```python
from build123d import *

# Parameters (mm, degrees)
F0_R     = 4
F0_W     = 8
F0_H     = 19
F1_DEPTH = 5
F0_H_2   = 1
F2_DEPTH = 8
F3_DEPTH = 5
F4_R     = 3
F5_SIZE2 = 2.99999
F5_SIZE  = 8.242422


# Not quite as in the source:
# - a fillet or chamfer is up to 0.001 mm smaller than in the source, because OpenCascade refuses the exact size


with BuildPart() as f1:
    # F0 (on Top) → F1 (new body)
    with BuildSketch(Plane.XY):
        Polygon((-15, 20), (-15, -25), (15, -25), (15, 20), (4, 20), (4, 1), (-4, 1), (-4, 20), align=None)
        with Locations((0, -15)):
            Circle(F0_R, mode=Mode.SUBTRACT)
        with Locations((0, 10.5)):
            Rectangle(F0_W, F0_H)
        with BuildLine():
            Line((-15, 25), (-15, 20))
            Line((-15, 20), (-4, 20))
            Line((-4, 20), (-4, 21))
            Line((-4, 21), (4, 21))
            Line((4, 21), (4, 20))
            Line((4, 20), (15, 20))
            Line((15, 20), (15, 25))
            Line((15, 25), (15, 31.3397459622))
            Line((15, 31.3397459622), (7.5, 27.0096189432))
            ThreePointArc((7.5, 27.0096189432), (0, 25), (-7.5, 27.0096189432))
            Line((-7.5, 27.0096189432), (-15, 31.3397459622))
            Line((-15, 31.3397459622), (-15, 25))
        make_face()
    extrude(amount=F1_DEPTH)

    # F0 (on Top) → F2 (join)
    with BuildSketch(Plane.XY):
        with Locations((0, 20.5)):
            Rectangle(F0_W, F0_H_2)
        with BuildLine():
            Line((-15, 25), (-15, 20))
            Line((-15, 20), (-4, 20))
            Line((-4, 20), (-4, 21))
            Line((-4, 21), (4, 21))
            Line((4, 21), (4, 20))
            Line((4, 20), (15, 20))
            Line((15, 20), (15, 25))
            Line((15, 25), (15, 31.3397459622))
            Line((15, 31.3397459622), (7.5, 27.0096189432))
            ThreePointArc((7.5, 27.0096189432), (0, 25), (-7.5, 27.0096189432))
            Line((-7.5, 27.0096189432), (-15, 31.3397459622))
            Line((-15, 31.3397459622), (-15, 25))
        make_face()
    extrude(amount=F2_DEPTH)

    # F0 (on Top) → F3 (join)
    with BuildSketch(Plane.XY):
        with Locations((0, 10.5)):
            Rectangle(F0_W, F0_H)
    extrude(amount=-F3_DEPTH)

    # F4
    f4_edges = [f1.edges().sort_by_distance(p)[0] for p in [
        (-15, 31.339746, 4),
        (15, 31.339746, 4),
        (-15, -25, 2.5),
        (15, -25, 2.5),
    ]]
    fillet(f4_edges, radius=F4_R)

    # F5 (size 8.2424322584 and 3 in the source; OpenCascade refuses exactly that, so slightly less here)
    f5_edges = [f1.edges().sort_by_distance(p)[0] for p in [
        (0, 20, 5),
    ]]
    f5_side = f1.faces().sort_by_distance((0, -1.950066, 5))[0]
    chamfer(f5_edges, length=F5_SIZE, length2=F5_SIZE2, reference=f5_side)


solid = f1.part
```
Geometry: final body of the model. Coordinates: model frame, mm. A direction names the side the tool comes from. Give positions to 0.01 mm unless a question says otherwise; leave off trailing zeros. Loops run counter-clockwise (first coordinate to the right, second up) from the corner with the lowest first, then second, coordinate; pieces in that order, holes last. Notation, with made-up numbers: (80, -7.5) -> (98, -7.5) arc R12 ccw to (98, 2.5) -> close; hole circle Ø9 at (15, 72). An arc over 180 degrees is marked (long way). Return JSON: item names as keys, results as strings.
Item 1: Section D-D, the plane y = 16. Output: boundary loops of the cut face in (x, z), plus the area to 3 significant figures.
Filled in:
{"outline": "(-15, 0) -> (-4, 0) -> (-4, -5) -> (4, -5) -> (4, 0) -> (15, 0) -> (15, 6.54) -> (-15, 6.54) -> close", "area": "236 mm^2"}
Item 2: Line query: line 1 (Y direction, x = 0, z = 1); line 2 (Z direction, x = -2.25, y = 23.5); line 3 (X direction, y = 15.5, z = -1.5). Output: solid intervals per line, ascending.
Filled in:
{"line 1": "-25 to -19, -11 to 25", "line 2": "0 to 8", "line 3": "-4 to 4"}
Item 3: Section B-B, the plane y = -15. Output: boundary loops of the cut face in (x, z).
Filled in:
{"outline": "(-15, 0) -> (-4, 0) -> (-4, 5) -> (-15, 5) -> close; (4, 0) -> (15, 0) -> (15, 5) -> (4, 5) -> close"}
Item 4: Pin query (flat end, axial travel): P1, Ø9, axis at x = 0, y = -15, coming from the +Z side; P2, Ø1.5, axis at x = -2.5, y = 22, coming from the -Z side; P3, Ø2.5, axis at x = -2, z = -3, coming from the +Y side. Return the tip coordinate at first contact, or that it passes through.
Filled in:
{"P1": "z = 5", "P2": "z = 0", "P3": "y = 20"}
Item 5: Access query for faces 5 (the flat face through (-4, 10, -2)), 6 (the flat face through (-8.979, 27.864, 3.944)), 7 (the flat face through (0, -6, 5)), 8 (the cylindrical face through (14.1, -24.14, 2.54)), 9 (the flat face through (0, 20, -2)). Directions: +Z, -Z, +X, -X, +Y, -Y. A direction counts if a zero-diameter tool reaches every point of the face in a straight line with its end or side. Return the directions, or none.
Filled in:
{"face 5": "-Z, -X, +Y, -Y", "face 6": "+Z, -Z, +Y", "face 7": "+Z, +X, -X, -Y", "face 8": "+Z, -Z, +X, -Y", "face 9": "-Z, +X, -X, +Y"}
Item 6: Mould query, pull axis X, two halves, no side actions, for faces 1 (the flat face through (15, 2, 3)), 2 (the flat face through (0, -4, 0)), 3 (the cylindrical face through (0, 25, 4)), 4 (the flat face through (9.021, 27.888, 3.944)). Classes: released by +X, released by -X, zero draft, split by the parting line, or undercut.
Filled in:
{"face 1": "released by +X", "face 2": "zero draft", "face 3": "undercut", "face 4": "undercut"}
Item 7: Section C-C, the plane z = 3.25. Output: boundary loops of the cut face in (x, y).
Filled in:
{"outline": "(-15, -22) arc R3 ccw to (-12, -25) -> (12, -25) arc R3 ccw to (15, -22) -> (15, 26.14) arc R3 ccw to (10.5, 28.74) -> (7.5, 27.01) arc R15 cw to (-7.5, 27.01) -> (-10.5, 28.74) arc R3 ccw to (-15, 26.14) -> close; hole circle Ø8 at (0, -15)"}
